Model file for the job. Use its own axes, mm. Face numbers are marked on the shaded views. A direction names the side the tool comes from. Round coordinates to 2 decimals unless told otherwise and drop trailing zeros. Loops run counter-clockwise (first coordinate to the right, second up) from the corner with the lowest first, then second, coordinate; pieces in that order, holes last. Notation, with made-up numbers: (62, 11.25) -> (92, 11.25) arc R29 cw to (92, 43.25) -> close; hole circle Ø7 at (46.25, -5). An arc over 180 degrees is marked (long way). Use a Markdown table: item, result.
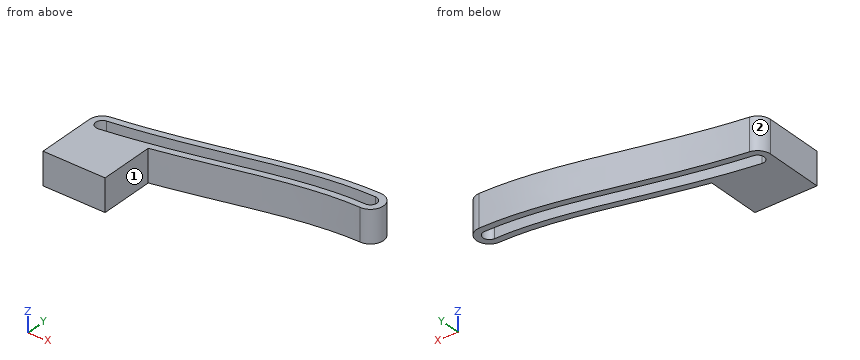
from build123d import *

# Parameters (mm, degrees)
BOSS_EXTRUDE1_DEPTH = 5
BOSS_EXTRUDE2_DEPTH = 5


with BuildPart() as part:
    # Sketch1 → Boss-Extrude1 (new body)
    with BuildSketch(Plane.XY):
        with BuildLine():
            add(Edge.make_bspline(
                [(28.284271497, 14), (26.832248759, 13.999999819), (23.942322546, 13.818389143), (18.107055454, 12.906300241), (10.807723253, 11.057558996), (1.886546527, 8.727754338), (-4.221907722, 7.524457078), (-7.287402613, 7.062387403)],
                knots=[0, 0, 0, 0, 0.085588552, 0.171177105, 0.342354209, 0.513531314, 0.684708419, 0.684708419, 0.684708419, 0.684708419], degree=3))
            ThreePointArc((-7.287402613, 7.062387403), (-9.563159868, 8.741949524), (-7.883597747, 11.017706779))
            add(Edge.make_bspline(
                [(28.284270998, 18), (26.686938926, 17.999999801), (23.476167151, 17.798108662), (17.246191739, 16.817667516), (9.748762966, 14.913893444), (0.95977161, 12.622104017), (-4.916957068, 11.464875912), (-7.883597747, 11.017706779)],
                knots=[0, 0, 0, 0, 0.085588552, 0.171177105, 0.342354209, 0.513531314, 0.684708419, 0.684708419, 0.684708419, 0.684708419], degree=3))
            ThreePointArc((28.284270998, 18), (30.284271247, 16.00000025), (28.284271497, 14))
        make_face()
        with BuildLine():
            ThreePointArc((28.284271123, 17), (29.284271247, 16.000000125), (28.284271372, 15))
            add(Edge.make_bspline(
                [(28.284271372, 15), (25.299991519, 14.999999628), (19.368041064, 14.256121216), (10.541251955, 12.021782806), (1.655347435, 9.701301701), (-4.395670061, 8.509561786), (-7.436451397, 8.051217247)],
                knots=[0, 0, 0, 0, 0.171177105, 0.342354209, 0.513531314, 0.684708419, 0.684708419, 0.684708419, 0.684708419], degree=3))
            ThreePointArc((-7.436451397, 8.051217247), (-8.574330024, 8.890998308), (-7.734548963, 10.028876935))
            add(Edge.make_bspline(
                [(28.284271123, 17), (26.723266395, 16.999999805), (23.592705995, 16.803178782), (17.46140767, 15.839825697), (10.013503037, 13.949809832), (1.19146534, 11.648516598), (-4.743194733, 10.479771203), (-7.734548963, 10.028876935)],
                knots=[0, 0, 0, 0, 0.085588552, 0.171177105, 0.342354209, 0.513531314, 0.684708419, 0.684708419, 0.684708419, 0.684708419], degree=3))
        make_face(mode=Mode.SUBTRACT)
    extrude(amount=BOSS_EXTRUDE1_DEPTH)

    # Sketch2 → Boss-Extrude2 (add)
    with BuildSketch(Plane.XY):
        with BuildLine():
            Line((-9.58550018, 0), (0, 0))
            Line((0, 0), (0, 8.405502806))
            add(Edge.make_bspline(
                [(0, 8.405502806), (-2.412231278, 7.886824896), (-4.846244229, 7.430349282), (-7.287402613, 7.062387403)],
                knots=[0.548394238, 0.548394238, 0.548394238, 0.548394238, 0.684708419, 0.684708419, 0.684708419, 0.684708419], degree=3))
            ThreePointArc((-7.287402613, 7.062387403), (-8.890070007, 7.524099346), (-9.58550018, 9.040047091))
            Line((-9.58550018, 9.040047091), (-9.58550018, 0))
        make_face()
    extrude(amount=BOSS_EXTRUDE2_DEPTH)


solid = part.part
Q1. Drill centre lines: L1, parallel to X at y = 4, z = 0.4; L2, parallel to Y at x = -5, z = 0.35; L3, parallel to Y at x = -2.5, z = 0.8. Where is each one in solid material? Low to high. Write a range as from..to.
Results list:
| item | result |
|---|---|
| L1 | x = -9.59..0 |
| L2 | y = 0..8.45, 10.48..11.49 |
| L3 | y = 0..8.91, 10.95..11.97 |
Q2. Tool access for the marked faces 1 and 2: list every direction of +Z, -Z, +X, -X, +Y, -Y with a clear straight run to the whole face (end or side of a thin tool).
Results list:
| item | result |
|---|---|
| face 1 | +Z, -Z, +X, -Y |
| face 2 | +Z, -Z, -X, +Y |
Q3. Band-saw the part on A-A, the plane y = 4.75. Give the cut face in (x, z).
Results list:
| item | result |
|---|---|
| outline | (-9.59, 0) -> (0, 0) -> (0, 5) -> (-9.59, 5) -> close |
Q4. Flat gauge pins, fed straight in: pin 1 (2 mm diameter, centred on y = 14, z = 2, fed in from +X); pin 2 (1.5 mm diameter, centred on x = 6.5, z = 1.5, fed in from -Y); pin 3 (2.5 mm diameter, centred on y = 2.5, z = 3, fed in from +X). Where does each tip first touch, or does it go through?
Results list:
| item | result |
|---|---|
| pin 1 | stops at x = 30.02 |
| pin 2 | stops at y = 9.75 |
| pin 3 | stops at x = 0 |
